The listing builds one solid part. Answer for the finished solid, in the listing's coordinates (mm). A direction names the side the tool comes from. Coordinates: 2 decimals unless noted, no trailing zeros. Order: outer loops, then holes, each group sorted by start corner. A loop starts at its lowest first (then second) coordinate and runs counter-clockwise, first axis right, second up. Notation, with made-up numbers: (63.5, 63.25) -> (86.5, 63.25) arc R20 cw to (86.5, 84.25) -> close; hole circle Ø11 at (57, -29.75). An arc over 180 degrees is marked (long way). Return JSON: item names as keys, results as strings.
Autodesk Inventor part; units mm, degrees
ref_plane "YZ Plane" through (0, 0, 0) normal (1, 0, 0) x (0, 1, 0)
ref_plane "XZ Plane" through (0, 0, 0) normal (0, 1, 0) x (-1, 0, 0)
ref_plane "XY Plane" through (0, 0, 0) normal (0, 0, 1) x (1, 0, 0)
sketch "Sketch1" plane through (0, 0, 0) normal (0, 1, 0) x (-1, 0, 0)
  circle A0 centre (-26.1551, -3.0475) radius 2.3
  arc A1 (-34.9051, -0.0475) -> (-17.4051, -0.0475) centre (-26.1551, -0.0475) ccw
  arc A2 (17.5949, -0.0475) -> (35.0949, -0.0475) centre (26.3449, -0.0475) ccw
  circle A3 centre (26.3449, -3.0475) radius 2.3
  circle A4 centre (-26.1551, -3.0475) radius 2.3
  circle A5 centre (26.3449, -3.0475) radius 2.3
  circle A6 centre (26.3449, -0.0475) radius 8.75
  circle A7 centre (-26.1551, -0.0475) radius 8.75
  line L0 (-34.9051, -0.0475) -> (-17.4051, -0.0475)
  line L1 (17.5949, -0.0475) -> (35.0949, -0.0475)
  circle A8 centre (-26.1551, -3.0475) radius 5.5
  circle A9 centre (26.3449, -3.0475) radius 5.5
  line L2 (-26.1551, -8.5475) -> (26.3449, -8.5475)
  line L3 (-26.1551, 2.4525) -> (26.3449, 2.4525)
  point P0 (0, 0)
  dimension "d0" = 11
  dimension "d1" = 11
  dimension "d41" = 4.6
  dimension "d42" = 4.6
extrude "Extrusion1" add sketch "Sketch1" along normal blind 10 contours L2 A8 L0 A1 | A1 A7 L3 A6 A2 L2 | A7 L0 A8 L3 | A8 L0 | L0 A8 | A2 L1 A9 L2 | L3 A9 L1 A6 | A9 L1 | A9 L1 picked at (-18.6939, -1.0014) picked at (-20.5799, 1.133) picked at (18.8536, -1.0809) picked at (20.7697, 1.133)
sketch "Sketch2" plane through (0, 10, 0) normal (0, 1, 0) x (1, 0, 0)
  line L0 (26.1551, 8.5475) -> (-26.3449, 8.5475)
  line L1 (-26.3449, -2.4525) -> (26.1551, -2.4525)
  arc A0 (-26.3449, 8.5475) -> (-26.3449, -2.4525) centre (-26.3449, 3.0475) ccw
  arc A1 (26.1551, -2.4525) -> (26.1551, 8.5475) centre (26.1551, 3.0475) ccw
  line L2 (-31.8449, 3.0475) -> (31.6551, 3.0475)
  line L3 (13.4051, -3.4525) -> (-13.5949, -3.4525)
  line L4 (-13.5949, -3.4525) -> (-13.5949, 9.5475)
  line L5 (-13.5949, 9.5475) -> (13.4051, 9.5475)
  line L6 (13.4051, 9.5475) -> (13.4051, -3.4525)
  line L7 (13.4051, -3.4525) -> (-13.5949, 9.5475) construction
  line L8 (-13.5949, -3.4525) -> (13.4051, 9.5475) construction
  point P0 (0, 0)
  point P1 (-0.0949, 3.0475)
  dimension "d4" = 27
  dimension "d5" = 13
extrude "Extrusion2" add sketch "Sketch2" along normal blind 14.56 contours L6 L2 L4 L0 | L0 L4 L5 L6 | L6 L1 L4 L2 | L6 L3 L4 L1
fillet "Fillet1" radius 2 2 edges at (-0.0949, 10, 3.4525) (-0.0949, 10, -9.5475)
sketch "Sketch3" plane through (0, 24.56, 0) normal (0, 1, 0) x (1, 0, 0)
  arc A0 (-6.4637, 1.2055) -> (-3.8927, 1.3299) centre (-5.0949, -0.4525) ccw
  arc A1 (3.5363, 1.2055) -> (6.1073, 1.3299) centre (4.9051, -0.4525) ccw
  circle A2 centre (4.9051, -0.4525) radius 2.15
  circle A3 centre (-5.0949, -0.4525) radius 2.15
  line L0 (-13.5949, 9.5475) -> (-13.5949, -3.4525)
  line L1 (13.4051, 9.5475) -> (-13.5949, 9.5475)
  line L2 (-13.5949, -3.4525) -> (13.4051, -3.4525)
  line L3 (13.4051, -3.4525) -> (13.4051, 9.5475)
  point P0 (0, 0)
  point P1 (6.1073, 1.3299)
  point P2 (3.5363, 1.2055)
  point P3 (-3.8927, 1.3299)
  point P4 (-6.4637, 1.2055)
  dimension "d12" = 8.5
  dimension "d13" = 8.5
  dimension "d43" = 2.15
  dimension "d44" = 2.15
extrude "Extrusion3" cut sketch "Sketch3" against normal blind 10 contours A3 A0 | A2 A1
sketch "Sketch4" plane through (0, 24.56, 0) normal (0, 1, 0) x (1, 0, 0)
  line L0 (13.4051, 9.5475) -> (-13.5949, 9.5475)
  line L1 (-13.5949, -2.4525) -> (-13.5949, 8.5475)
  line L2 (13.4051, 9.5475) -> (-13.5949, 9.5475)
  line L3 (-13.5949, 9.5475) -> (-13.5949, 3.0475)
  line L4 (-13.5949, 3.0475) -> (13.4051, 3.0475)
  line L5 (13.4051, 3.0475) -> (13.4051, 9.5475)
  point P0 (0, 0)
extrude "Extrusion4" cut sketch "Sketch4" against normal blind 4.2875
fillet "Fillet2" radius 6.7625 1 edges at (-0.0949, 20.2725, -9.5475)
sketch "Sketch5" plane through (0, 24.56, 0) normal (0, 1, 0) x (1, 0, 0)
  line L0 (-13.5949, -3.4525) -> (13.4051, -3.4525)
  line L1 (-10.3949, -3.4525) -> (-10.3949, -67.4525)
  line L2 (10.2051, -3.4525) -> (10.2051, -67.4525)
  line L3 (-13.5949, 3.0475) -> (-13.5949, -3.4525)
  circle A0 centre (-5.0949, -49.4525) radius 2.15
  line L4 (13.4051, -3.4525) -> (13.4051, 3.0475)
  circle A1 centre (4.9051, -49.4525) radius 2.15
  circle A2 centre (4.9051, -49.4525) radius 3
  circle A3 centre (-5.0949, -49.4525) radius 3
  line L5 (-10.3949, -67.4525) -> (10.2051, -67.4525)
  line L6 (-10.3949, -67.4525) -> (-13.5949, -67.4525)
  line L7 (-13.5949, -67.4525) -> (-13.5949, -3.4525)
  line L8 (10.2051, -67.4525) -> (13.4051, -67.4525)
  line L9 (13.4051, -67.4525) -> (13.4051, -3.4525)
  line L10 (-5.0949, -46.4525) -> (4.9051, -46.4525)
  line L11 (10.2051, -46.4525) -> (-10.3949, -46.4525)
  line L12 (-0.65, -46.4525) -> (-0.65, -51.4525)
  line L13 (-0.65, -51.4525) -> (0.65, -51.4525)
  line L14 (0.65, -51.4525) -> (0.65, -46.4525)
  line L15 (0, -46.4525) -> (-0.65, -51.4525) construction
  line L16 (0, -46.4525) -> (0.65, -51.4525) construction
  point P0 (0, 0)
  point P1 (13.4051, -0.2025)
  point P2 (4.9051, -46.4525)
  dimension "d28" = 6
  dimension "d29" = 6
  dimension "d19" = 3.2
  dimension "d20" = 64
  dimension "d21" = 3.2
  dimension "d22" = 64
  dimension "d23" = 46
  dimension "d24" = 8.5
  dimension "d25" = 4.3
  dimension "d26" = 8.5
  dimension "d27" = 4.3
  dimension "d30" = 1.3
extrude "Extrusion5" add sketch "Sketch5" against normal blind 4.2875 contours L0 L1 L6 L7 | L0 L9 L8 L2 | A2 | A3 | L11 L10 L12 L13 L14 L2 L5 L1
sketch "Sketch6" plane through (0, 24.56, 0) normal (0, 1, 0) x (1, 0, 0)
  line L0 (13.4051, -67.4525) -> (-13.5949, -67.4525)
  line L1 (-13.5949, -67.4525) -> (13.4051, -67.4525)
  line L2 (13.4051, -67.4525) -> (13.4051, -78.4525)
  line L3 (13.4051, -78.4525) -> (-13.5949, -78.4525)
  line L4 (-13.5949, -78.4525) -> (-13.5949, -67.4525)
  circle A0 centre (26.1551, 3.0475) radius 2.3
  circle A1 centre (-26.3449, 3.0475) radius 2.3
  point P0 (0, 0)
  dimension "d34" = 11
extrude "Extrusion6" add sketch "Sketch6" against normal up to surface (14.56 mm away) contours L2 L3 L4 L0
ref_plane "Work Plane1" through (-13.5949, 24.56, 34.9525) normal (0, 0, 1) x (1, 0, 0)
sketch "Sketch7" plane through (0, 24.56, 0) normal (0, 1, 0) x (1, 0, 0)
  point P0 (0, 0)
mirror "Mirror1" about plane through (-13.5949, 24.56, 34.9525) normal (0, 0, 1) of "Extrusion1"
sketch "Sketch8" plane through (0, 24.56, 0) normal (0, 1, 0) x (1, 0, 0)
  line L0 (0.6, -3.9565) -> (-0.6, -3.9565)
  line L1 (-0.6, -3.9565) -> (-0.6, 3.9565)
  line L2 (-0.6, 3.9565) -> (0.6, 3.9565)
  line L3 (0.6, 3.9565) -> (0.6, -3.9565)
  line L4 (0.6, -3.9565) -> (-0.6, 3.9565) construction
  line L5 (-0.6, -3.9565) -> (0.6, 3.9565) construction
  point P0 (0, 0)
  dimension "d38" = 1.2
extrude "Extrusion7" cut sketch "Sketch8" against normal blind 4
properties part number "SERVO_MOUNT_TOBASE"
Item 1: Flat-ended cylindrical pins translate along their axes: pin 1 (2 mm diameter, centred on x = 13.5, z = 51, fed in from -Y); pin 2 (7.5 mm diameter, centred on y = 19, z = 54.5, fed in from +X); pin 3 (5 mm diameter, centred on x = 8, y = 16.5, fed in from -Z). Find the tip coordinate at first contact, or state that the pin passes through.
Answer list:
{"pin 1": "y = 20.27", "pin 2": "x = 13.41", "pin 3": "z = -9.53"}
Item 2: The part is cut by section A-A on x = 20.5. Determine the outline of the cut face in (y, z).
Answer list:
{"outline": "(0, -8.55) -> (10, -8.55) -> (10, 2.45) -> (0, 2.45) -> close; (0, 67.45) -> (10, 67.45) -> (10, 78.45) -> (0, 78.45) -> close"}
Item 3: The part is cut by section D-D on y = 19. Determine the outline of the cut face in (x, z), plus the area to 3 significant figures.
Answer list:
{"outline": "(-13.59, -6.73) -> (13.41, -6.73) -> (13.41, 3.45) -> (-13.59, 3.45) -> close; (-13.59, 67.45) -> (13.41, 67.45) -> (13.41, 78.45) -> (-13.59, 78.45) -> close; hole (-6.46, -1.21) arc R2.15 ccw to (-3.89, -1.33) arc R2.15 ccw (long way) to start; hole (3.54, -1.21) arc R2.15 ccw to (6.11, -1.33) arc R2.15 ccw (long way) to start", "area": "543 mm2"}
Item 4: Which of the six approach directions +Z, -Z, +X, -X, +Y, -Y give full straight-line access (tool end or side, diameter ignored) to faces 1 (the flat face through (0, 5, -8.548)), 2 (the flat face through (0, 18, 3.452)), 3 (the flat face through (0, 5, 2.452)), 4 (the flat face through (-5, 22, 46.452))?
Answer list:
{"face 1": "-Z, +X, -X, -Y", "face 2": "-Y", "face 3": "+X, -X, -Y", "face 4": "+Y, -Y"}
Item 5: The part is cut by section B-B on y = 6.75. Determine the outline of the cut face in (x, z), plus the area to 3 significant figures.
Answer list:
{"outline": "(-26.34, -8.55) -> (26.16, -8.55) arc R5.5 ccw to (26.16, 2.45) -> (-26.34, 2.45) arc R5.5 ccw to start; (-26.34, 67.45) -> (26.16, 67.45) arc R5.5 ccw to (26.16, 78.45) -> (-26.34, 78.45) arc R5.5 ccw to start; hole circle Ø4.6 at (-26.34, -3.05); hole circle Ø4.6 at (-26.34, 72.95); hole circle Ø4.6 at (26.16, -3.05); hole circle Ø4.6 at (26.16, 72.95)", "area": "1,280 mm2"}
Item 6: Determine the mould class of faces 5 (the flat face through (-5, 14.56, 0)), 6 (the cylindrical face through (31.654, 4.93, -3.168)), 7 (the flat face through (-23, 10, 73)) for opening direction X: pulls with the +X half, pulls with the -X half, needs draft (parallel to the pull), parting line crosses it, or undercut.
Answer list:
{"face 5": "undercut", "face 6": "pulls with the +X half", "face 7": "needs draft"}
Item 7: Find the intervals of material crossed by probe 1 along Z at (x, y) = (10.5, 1); probe 2 along Z at (x, y) = (7, 12.5); probe 3 along X at (y, z) = (22.5, 62), in increasing order.
Answer list:
{"probe 1": "-8.55 to 2.45, 67.45 to 78.45", "probe 2": "-9.55 to 3.45, 67.45 to 78.45", "probe 3": "-13.59 to 13.41"}
Item 8: The part is cut by section C-C on z = 15. Determine the outline of the cut face in (x, y).
Answer list:
{"outline": "(-13.59, 20.27) -> (-10.39, 20.27) -> (-10.39, 24.56) -> (-13.59, 24.56) -> close; (10.21, 20.27) -> (13.41, 20.27) -> (13.41, 24.56) -> (10.21, 24.56) -> close"}
